Geometry: final body of the model. Coordinates: model frame, mm. A direction names the side the tool comes from. Coordinates: 2 decimals unless noted, no trailing zeros. Order: outer loops, then holes, each group sorted by start corner. A loop starts at its lowest first (then second) coordinate and runs counter-clockwise, first axis right, second up. Notation, with made-up numbers: M 17,-28.5 L 76,-28.5 A20 ccw 76,-7.5 Z; hole C 60.25,31.25 d9. An arc over 180 degrees is marked long. One line per question, with ' | ' between items.
from build123d import *

# Parameters (mm, degrees)
SKETCH2_R           = 27
SKETCH2_R_2         = 2
BOSS_EXTRUDE1_DEPTH = 4


with BuildPart() as part:
    # Sketch2 → Boss-Extrude1 (new body)
    with BuildSketch(Plane.XY):
        Circle(SKETCH2_R)
        with Locations((24, 0)):
            Circle(SKETCH2_R_2, mode=Mode.SUBTRACT)
        with BuildLine():
            Line((-2, 18.574175621), (-2, 6))
            ThreePointArc((-2, 6), (-3.171572875, 3.171572875), (-6, 2))
            Line((-6, 2), (-18.574175621, 2))
            ThreePointArc((-18.574175621, 2), (-20.130148831, 2.743438275), (-20.529352002, 4.421052632))
            ThreePointArc((-20.529352002, 4.421052632), (-14.849242405, 14.849242405), (-4.421052632, 20.529352002))
            ThreePointArc((-4.421052632, 20.529352002), (-2.743438275, 20.130148831), (-2, 18.574175621))
        make_face(mode=Mode.SUBTRACT)
        with BuildLine():
            Line((18.574175621, 2), (6, 2))
            ThreePointArc((6, 2), (3.171572875, 3.171572875), (2, 6))
            Line((2, 6), (2, 18.574175621))
            ThreePointArc((2, 18.574175621), (2.743438275, 20.130148831), (4.421052632, 20.529352002))
            ThreePointArc((4.421052632, 20.529352002), (14.849242405, 14.849242405), (20.529352002, 4.421052632))
            ThreePointArc((20.529352002, 4.421052632), (20.130148831, 2.743438275), (18.574175621, 2))
        make_face(mode=Mode.SUBTRACT)
        with BuildLine():
            Line((18.574175621, -2), (6, -2))
            ThreePointArc((6, -2), (3.171572875, -3.171572875), (2, -6))
            Line((2, -6), (2, -18.574175621))
            ThreePointArc((2, -18.574175621), (2.743438275, -20.130148831), (4.421052632, -20.529352002))
            ThreePointArc((4.421052632, -20.529352002), (14.849242405, -14.849242405), (20.529352002, -4.421052632))
            ThreePointArc((20.529352002, -4.421052632), (20.130148831, -2.743438275), (18.574175621, -2))
        make_face(mode=Mode.SUBTRACT)
        with BuildLine():
            Line((-6, -2), (-18.574175621, -2))
            ThreePointArc((-18.574175621, -2), (-20.130148831, -2.743438275), (-20.529352002, -4.421052632))
            ThreePointArc((-20.529352002, -4.421052632), (-14.849242405, -14.849242405), (-4.421052632, -20.529352002))
            ThreePointArc((-4.421052632, -20.529352002), (-2.743438275, -20.130148831), (-2, -18.574175621))
            Line((-2, -18.574175621), (-2, -6))
            ThreePointArc((-2, -6), (-3.171572875, -3.171572875), (-6, -2))
        make_face(mode=Mode.SUBTRACT)
    extrude(amount=BOSS_EXTRUDE1_DEPTH)


solid = part.part
1. Access query for faces 1 (the face through (0, 0, 0)), 2 (the face through (-14.97, -14.73, 1.97)). Directions: +Z, -Z, +X, -X, +Y, -Y. A direction counts if a zero-diameter tool reaches every point of the face in a straight line with its end or side. Return the directions, or none.
Response values:
face 1: -Z, +X, -X, +Y, -Y | face 2: +Z, -Z
2. Section D-D, the plane y = 0. Output: boundary loops of the cut face in (x, z).
Response values:
outline: M -27,0 L 22,0 L 22,4 L -27,4 Z; M 26,0 L 27,0 L 27,4 L 26,4 Z
3. Section B-B, the plane x = 3.5. Output: boundary loops of the cut face in (y, z).
Response values:
outline: M -26.77,0 L -20.51,0 L -20.51,4 L -26.77,4 Z; M -2.88,0 L 2.88,0 L 2.88,4 L -2.88,4 Z; M 20.51,0 L 26.77,0 L 26.77,4 L 20.51,4 Z
4. Section C-C, the plane y = 8.5. Output: boundary loops of the cut face in (x, z), and give its area (3 significant figures).
Response values:
outline: M -25.63,0 L -19.2,0 L -19.2,4 L -25.63,4 Z; M -2,0 L 2,0 L 2,4 L -2,4 Z; M 19.2,0 L 25.63,0 L 25.63,4 L 19.2,4 Z | area: 67.4 mm^2
5. Section A-A, the plane z = 1.25. Output: boundary loops of the cut face in (x, y).
Response values:
outline: C 0,0 d54; hole M -20.53,-4.42 A21 ccw -4.42,-20.53 A2 ccw -2,-18.57 L -2,-6 A4 ccw -6,-2 L -18.57,-2 A2 ccw Z; hole M -20.53,4.42 A2 ccw -18.57,2 L -6,2 A4 ccw -2,6 L -2,18.57 A2 ccw -4.42,20.53 A21 ccw Z; hole M 2,-18.57 A2 ccw 4.42,-20.53 A21 ccw 20.53,-4.42 A2 ccw 18.57,-2 L 6,-2 A4 ccw 2,-6 Z; hole M 2,6 A4 ccw 6,2 L 18.57,2 A2 ccw 20.53,4.42 A21 ccw 4.42,20.53 A2 ccw 2,18.57 Z; hole C 24,0 d4
6. Draft query along X for faces 3 (the face through (0, 0, 4)), 4 (the face through (-2.763, -20.146, 1.972)). Return one class per face: pulls with the +X half, pulls with the -X half, needs draft (parallel to the pull), parting line crosses it, or undercut.
Response values:
face 3: needs draft | face 4: undercut
7. Material intervals for line 1 (Y direction, x = 4, z = 1.6); line 2 (Y direction, x = -14, z = 3); line 3 (X direction, y = -11.5, z = 3.1), sorted ascending. Write a range as [from, to].
Response values:
line 1: y = [-26.7, -20.57], [-2.54, 2.54], [20.57, 26.7] | line 2: y = [-23.09, -15.65], [-2, 2], [15.65, 23.09] | line 3: x = [-24.43, -17.57], [-2, 2], [17.57, 24.43]
8. Pin query (flat end, axial travel): P1, Ø2, axis at y = 11.5, z = 3, coming from the -X side; P2, Ø2, axis at x = 2, z = 3.5, coming from the +Y side; P3, Ø2, axis at x = 12.5, z = 2.5, coming from the -Y side. Return the tip coordinate at first contact, or that it passes through.
Response values:
P1: stops at x = -24.87 | P2: stops at y = 26.98 | P3: stops at y = -24.43
